```python
from build123d import *

# Parameters (mm, degrees)
BOX013_W     = 3
BOX013_H     = 3
BOX013_DEPTH = 10
BOX009_W     = 1
BOX009_H     = 3
BOX009_DEPTH = 3
BOX010_W     = 1
BOX010_H     = 3
BOX010_DEPTH = 3
BOX011_W     = 6
BOX011_H     = 1
BOX011_DEPTH = 3
BOX012_W     = 6
BOX012_H     = 1
BOX012_DEPTH = 3
BOX008_W     = 6
BOX008_H     = 3.5
BOX008_DEPTH = 20


with BuildPart() as box013:
    # Box013 → Box013 (new body)
    with BuildSketch(Plane(origin=(13.5, 19.25, 20), x_dir=(1, 0, 0), z_dir=(0, 0, 1))):
        with Locations((1.5, 1.5)):
            Rectangle(BOX013_W, BOX013_H)
    extrude(amount=BOX013_DEPTH)


with BuildPart() as box009:
    # Box009 → Box009 (new body)
    with BuildSketch(Plane(origin=(11, 7.25, 7), x_dir=(1, 0, 0), z_dir=(0, 0, 1))):
        with Locations((0.5, 1.5)):
            Rectangle(BOX009_W, BOX009_H)
    extrude(amount=BOX009_DEPTH)


with BuildPart() as box010:
    # Box010 → Box010 (new body)
    with BuildSketch(Plane(origin=(18, 7.25, 7), x_dir=(1, 0, 0), z_dir=(0, 0, 1))):
        with Locations((0.5, 1.5)):
            Rectangle(BOX010_W, BOX010_H)
    extrude(amount=BOX010_DEPTH)


with BuildPart() as box011:
    # Box011 → Box011 (new body)
    with BuildSketch(Plane(origin=(12, 6, 7), x_dir=(1, 0, 0), z_dir=(0, 0, 1))):
        with Locations((3, 0.5)):
            Rectangle(BOX011_W, BOX011_H)
    extrude(amount=BOX011_DEPTH)


with BuildPart() as box012:
    # Box012 → Box012 (new body)
    with BuildSketch(Plane(origin=(12, 10.5, 7), x_dir=(1, 0, 0), z_dir=(0, 0, 1))):
        with Locations((3, 0.5)):
            Rectangle(BOX012_W, BOX012_H)
    extrude(amount=BOX012_DEPTH)


with BuildPart() as bt_ex2:
    # Box008 → Box008 (new body)
    with BuildSketch(Plane(origin=(12, 7, 9), x_dir=(1, 0, 0), z_dir=(0, 0, 1))):
        with Locations((3, 1.75)):
            Rectangle(BOX008_W, BOX008_H)
    extrude(amount=BOX008_DEPTH)

    # Fusion001: union Box009, Box010, Box011, Box012
    add(box009.part)
    add(box010.part)
    add(box011.part)
    add(box012.part)


with BuildPart() as bt_ex2_1:
    # Fusion001 placement: moved
    add(bt_ex2.part.moved(Location((0, 12, 0))))

    # Fusion006: union Box013
    add(box013.part)


solid = bt_ex2_1.part
```
Here's how the part is built. I have some questions about the finished solid (model axes, mm). A direction names the side the tool comes from. Coordinates: 2 decimals unless noted, no trailing zeros. Loops run counter-clockwise (first coordinate to the right, second up) from the corner with the lowest first, then second, coordinate; pieces in that order, holes last. Notation, with made-up numbers: (4.5, -19) - (34.5, -19) arc R22 cw to (34.5, -13) - close; hole circle Ø6 at (-21, 40). An arc over 180 degrees is marked (long way). Return JSON: item names as keys, results as strings. Group by question number.
Item 1: Will these pins go through, and if not, where does the flat tip stop? P1, Ø3, axis at y = 19, z = 14.5, coming from the -X side; P2, Ø0.5, axis at y = 20.5, z = 29.5, coming from the +X side; P3, Ø1.1, axis at x = 15.5, z = 29.5, coming from the +Y side; P4, Ø3, axis at x = 13.5, y = 20, coming from the -Z side.
Item 2: We'd pull the mould along X, two halves only. Please class faces 1 (the face through (15, 19, 19)), 2 (the face through (12, 21, 8)), 3 (the face through (11, 21, 8)): +X half, -X half, draft (parallel to the pull), parting line (faces both ways), or undercut.
Item 3: If we section it at D-D on x = 18.5: Write out the boundary of the cut face in (y, z), and give its area (3 significant figures).
Item 4: If we section it at C-C on z = 15.75: Write out the boundary of the cut face in (x, y).
Item 5: If we section it at A-A on y = 21.65: Write out the boundary of the cut face in (x, z), and give its area (3 significant figures).
Item 6: On a 3-axis mill with a long thin cutter (end or side, diameter ignored), from which of +Z, -Z, +X, -X, +Y, -Y can I reach the whole of each face in a straight line? I mean faces 4 (the face through (18.5, 20.8, 10)), 5 (the face through (13.5, 20.7, 29.5)), 6 (the face through (15, 22.25, 29.5)), 7 (the face through (15, 19, 8)), 8 (the face through (15, 21, 9)). Say none if no direction works.
Item 7: I need wall thicknesses on line 1 (Z direction, x = 14.75, y = 20.6); line 2 (Y direction, x = 15.5, z = 16.25); line 3 (Z direction, x = 15, y = 18.8). Which ranges of each line are inside material? Lowest first, please. Write a range as from..to.
Item 8: If we section it at B-B on x = 15.75: Write out the boundary of the cut face in (y, z), and give its area (3 significant figures).
Calculated:
{
 "1": {"P1": "stops at x = 12", "P2": "stops at x = 16.5", "P3": "stops at y = 22.5", "P4": "stops at z = 7"},
 "2": {"face 1": "draft", "face 2": "undercut", "face 3": "-X half"},
 "3": {"outline": "(19.25, 7) - (22.25, 7) - (22.25, 10) - (19.25, 10) - close", "area": "9.00 mm^2"},
 "4": {"outline": "(12, 19) - (18, 19) - (18, 22.5) - (12, 22.5) - close"},
 "5": {"outline": "(11, 7) - (12, 7) - (12, 9) - (18, 9) - (18, 7) - (19, 7) - (19, 10) - (18, 10) - (18, 29) - (16.5, 29) - (16.5, 30) - (13.5, 30) - (13.5, 29) - (12, 29) - (12, 10) - (11, 10) - close", "area": "129 mm^2"},
 "6": {"face 4": "+Z, +X, +Y, -Y", "face 5": "+Z, -X, +Y, -Y", "face 6": "+Z, +X, -X, +Y", "face 7": "-Z, +X, -X", "face 8": "-Z"},
 "7": {"line 1": "z = 9..30", "line 2": "y = 19..22.5", "line 3": "z = 7..10"},
 "8": {"outline": "(18, 7) - (19, 7) - (19, 9) - (22.5, 9) - (22.5, 7) - (23.5, 7) - (23.5, 10) - (22.5, 10) - (22.5, 29) - (22.25, 29) - (22.25, 30) - (19.25, 30) - (19.25, 29) - (19, 29) - (19, 10) - (18, 10) - close", "area": "79.0 mm^2"}
}
